from build123d import *

# Parameters (mm, degrees)
SKETCH1_R           = 0.5
BOSS_EXTRUDE1_DEPTH = 2.5
SKETCH2_R           = 0.75
CUT_EXTRUDE1_DEPTH  = 9
SKETCH3_R           = 2.7
SKETCH3_R_2         = 2
BOSS_EXTRUDE2_DEPTH = 1.1


with BuildPart() as part:
    # Sketch1 → Boss-Extrude1 (new body)
    with BuildSketch(Plane(origin=(0, 0, 0), x_dir=(1, 0, 0), z_dir=(0, 1, 0))):
        with BuildLine():
            Line((0.594059406, 2.940594059), (20, 1))
            ThreePointArc((20, 1), (21, 0), (20, -1))
            Line((20, -1), (0.594059406, -2.940594059))
            ThreePointArc((0.594059406, -2.940594059), (0, -3), (-0.594059406, -2.940594059))
            Line((-0.594059406, -2.940594059), (-20, -1))
            ThreePointArc((-20, -1), (-21, 0), (-20, 1))
            Line((-20, 1), (-0.594059406, 2.940594059))
            ThreePointArc((-0.594059406, 2.940594059), (0, 3), (0.594059406, 2.940594059))
        make_face()
        with Locations(Location((5, 0, 0), (0, 0, 270))):
            Circle(SKETCH1_R, mode=Mode.SUBTRACT)
        with Locations(Location((10, 0, 0), (0, 0, 270))):
            Circle(SKETCH1_R, mode=Mode.SUBTRACT)
        with Locations(Location((15, 0, 0), (0, 0, 270))):
            Circle(SKETCH1_R, mode=Mode.SUBTRACT)
        with Locations(Location((20, 0, 0), (0, 0, 270))):
            Circle(SKETCH1_R, mode=Mode.SUBTRACT)
        with Locations(Location((-20, 0, 0), (0, 0, 90))):
            Circle(SKETCH1_R, mode=Mode.SUBTRACT)
        with Locations(Location((-15, 0, 0), (0, 0, 90))):
            Circle(SKETCH1_R, mode=Mode.SUBTRACT)
        with Locations(Location((-10, 0, 0), (0, 0, 90))):
            Circle(SKETCH1_R, mode=Mode.SUBTRACT)
        with Locations(Location((-5, 0, 0), (0, 0, 90))):
            Circle(SKETCH1_R, mode=Mode.SUBTRACT)
        with BuildLine():
            Line((-0.921954446, -0.6), (0.921954446, -0.6))
            ThreePointArc((0.921954446, -0.6), (0, 1.1), (-0.921954446, -0.6))
        make_face(mode=Mode.SUBTRACT)
    extrude(amount=BOSS_EXTRUDE1_DEPTH)

    # Sketch2 → Cut-Extrude1 (cut)
    with BuildSketch(Plane.XY):
        with Locations(Location((0, 1.25, 0), (0, 0, 180))):
            Circle(SKETCH2_R)
    extrude(amount=CUT_EXTRUDE1_DEPTH, mode=Mode.SUBTRACT)

    # Sketch3 → Boss-Extrude2 (add)
    with BuildSketch(Plane(origin=(0, 0, 0), x_dir=(1, 0, 0), z_dir=(0, 1, 0))):
        with Locations(Location((0, 0, 0), (0, 0, 270))):
            Circle(SKETCH3_R)
        with Locations(Location((0, 0, 0), (0, 0, 270))):
            Circle(SKETCH3_R_2, mode=Mode.SUBTRACT)
    extrude(amount=-BOSS_EXTRUDE2_DEPTH)


solid = part.part
Design review of the part built by this model. Coordinates are the model's own, in mm. A direction names the side the tool comes from. Coordinates: 2 decimals unless noted, no trailing zeros. Loops run counter-clockwise (first coordinate to the right, second up) from the corner with the lowest first, then second, coordinate; pieces in that order, holes last. Notation, with made-up numbers: (74.25, 24.25) - (129.25, 24.25) arc R22 ccw to (129.25, 60.25) - close; hole circle Ø6 at (33.25, 46.5). An arc over 180 degrees is marked (long way). Use CSV: the item, a comma, the result in double quotes. Start each with the question number.
1. For faces 4 (the cylindrical face through (15.496, 1.232, -0.065)), 5 (the cylindrical face through (0.098, 0.506, 1.783)), 6 (the flat face through (0, 0, 1)), list the 3-axis set-ups (+Z, -Z, +X, -X, +Y, -Y) from which the entire face can be reached by the end or side of a thin tool; tool diameter is ignored.
2. To check wall thickness, follow probe 1 along Z at (x, y) = (-20, 1.6); probe 2 along Y at (x, z) = (0, 1.55); probe 3 along Z at (x, y) = (-5, 0.6). State the ranges of each line that lie inside material, in increasing order.
3. Add section A-A on x = 0. Give the boundary of the cut face in (y, z).
4. Add section C-C on x = 10. Give the boundary of the cut face in (y, z).
5. Clearance check with flat-ended pins moving along their axes: pin 1 (2.5 mm diameter, centred on x = 0, z = 0, fed in from -Y); pin 2 (2 mm diameter, centred on x = 6, y = 1.5, fed in from +Z); pin 3 (2 mm diameter, centred on x = -11.5, y = 2, fed in from +Z). State where each tip first meets the part, or that it passes through.
6. Add section B-B on x = -15. Give the boundary of the cut face in (y, z).
7. Mouldability with a two-part tool opening along Z and no side actions: class faces 1 (the cylindrical face through (0, 1.2, -1.1)), 2 (the cylindrical face through (-21, 1, 0)), 3 (the flat face through (0, 2.5, 1)) as released by +Z, released by -Z, zero draft, split by the parting line, or undercut.
Resolved:
1,face 4,"+Y, -Y"
1,face 5,"+Z"
1,face 6,"-Y"
2,probe 1,"-1 to -0.5, 0.5 to 1"
2,probe 2,"0 to 0.5, 2 to 2.5"
2,probe 3,"-2.5 to -0.5, 0.5 to 2.5"
3,outline,"(-1.1, -2.7) - (0, -2.7) - (0, -3) - (2.5, -3) - (2.5, -1.1) - (0, -1.1) - (0, -2) - (-1.1, -2) - close; (-1.1, 2) - (0, 2) - (0, 0.6) - (0.5, 0.6) - (0.5, 3) - (0, 3) - (0, 2.7) - (-1.1, 2.7) - close; (2, 0.6) - (2.5, 0.6) - (2.5, 3) - (2, 3) - close"
4,outline,"(0, -2) - (2.5, -2) - (2.5, -0.5) - (0, -0.5) - close; (0, 0.5) - (2.5, 0.5) - (2.5, 2) - (0, 2) - close"
5,pin 1,"y = 0"
5,pin 2,"z = 2.5"
5,pin 3,"z = 1.95"
6,outline,"(0, -1.5) - (2.5, -1.5) - (2.5, -0.5) - (0, -0.5) - close; (0, 0.5) - (2.5, 0.5) - (2.5, 1.5) - (0, 1.5) - close"
7,face 1,"undercut"
7,face 2,"split by the parting line"
7,face 3,"zero draft"
